Geometry check sheet. Reference: the model listing, model coordinates, mm. Face numbers are marked on the shaded views. A direction names the side the tool comes from. Give positions to 0.01 mm unless a question says otherwise; leave off trailing zeros. Order: outer loops, then holes, each group sorted by start corner. A loop starts at its lowest first (then second) coordinate and runs counter-clockwise, first axis right, second up. Notation, with made-up numbers: (70.25, 83.25) - (77.25, 83.25) arc R28 ccw to (77.25, 105.25) - close; hole circle Ø1 at (6.25, 38.25). An arc over 180 degrees is marked (long way). Put each result on its own line as item: value. Start each with the question number.
```python
from build123d import *

# Parameters (mm, degrees)
F1_DEPTH    = 10
F3_DEPTH    = 1
F4_T1_DEPTH = 100
F4_T4_ANGLE = 180
F4_T6_ANGLE = 180
F6_DEPTH    = 9
F7_R        = 1.1168399156
F8_DEPTH    = 100


# Not quite as in the source:
# - a fillet or chamfer that OpenCascade refuses, or shapes differently, is made with other operations: its cross-section is extruded or revolved along the edge and cut away or added


with BuildPart() as f1:
    # F0 (on Top) → F1 (new body)
    with BuildSketch(Plane.XY):
        with BuildLine():
            Line((48.6515399069, 4.7592671573), (-51.3484600931, 4.7592671573))
            ThreePointArc((-51.3484600931, 4.7592671573), (-61.8484600931, -5.7407328427), (-51.3484600931, -16.2407328427))
            Line((-51.3484600931, -16.2407328427), (48.6515399069, -16.2407328427))
            ThreePointArc((48.6515399069, -16.2407328427), (59.1515399069, -5.7407328427), (48.6515399069, 4.7592671573))
        make_face()
    extrude(amount=F1_DEPTH)

    # F2 (on face) → F3 (join)
    with BuildSketch(Plane.XY.offset(10)):
        with BuildLine():
            Line((48.6515399069, 6.7592671573), (-51.3484600931, 6.7592671573))
            ThreePointArc((-51.3484600931, 6.7592671573), (-63.8484600931, -5.7407328427), (-51.3484600931, -18.2407328427))
            Line((-51.3484600931, -18.2407328427), (48.6515399069, -18.2407328427))
            ThreePointArc((48.6515399069, -18.2407328427), (61.1515399069, -5.7407328427), (48.6515399069, 6.7592671573))
        make_face()
        with BuildLine():
            Line((-51.3484600931, 4.7592671573), (48.6515399069, 4.7592671573))
            ThreePointArc((48.6515399069, 4.7592671573), (59.1515399069, -5.7407328427), (48.6515399069, -16.2407328427))
            Line((48.6515399069, -16.2407328427), (-51.3484600931, -16.2407328427))
            ThreePointArc((-51.3484600931, -16.2407328427), (-61.8484600931, -5.7407328427), (-51.3484600931, 4.7592671573))
        make_face(mode=Mode.SUBTRACT)
        with BuildLine():
            ThreePointArc((48.6515399069, -16.2407328427), (59.1515399069, -5.7407328427), (48.6515399069, 4.7592671573))
            Line((48.6515399069, 4.7592671573), (-51.3484600931, 4.7592671573))
            ThreePointArc((-51.3484600931, 4.7592671573), (-61.8484600931, -5.7407328427), (-51.3484600931, -16.2407328427))
            Line((-51.3484600931, -16.2407328427), (48.6515399069, -16.2407328427))
        make_face()
    extrude(amount=F3_DEPTH)

    # F4: fillet of radius 6 on 4 edges, made by hand

    # F4_s2 → F4_t1 (cut)
    with BuildSketch(Plane.YZ.offset(-51.3484600931)):
        with BuildLine():
            ThreePointArc((6.7592671573, 10), (5.1746931745, 10.7445626465), (3.4426423669, 11))
            Line((3.4426423669, 11), (6.7592671573, 11))
            Line((6.7592671573, 11), (6.7592671573, 10))
        make_face()
        with BuildLine():
            ThreePointArc((-18.2407328427, 10), (-16.6561588599, 10.7445626465), (-14.9241080524, 11))
            Line((-14.9241080524, 11), (-18.2407328427, 11))
            Line((-18.2407328427, 11), (-18.2407328427, 10))
        make_face()
    extrude(amount=F4_T1_DEPTH, mode=Mode.SUBTRACT)

    # F4_s3 → F4_t4 (revolve, cut)
    with BuildSketch(Plane.YZ.offset(48.6515399069)):
        with BuildLine():
            ThreePointArc((-18.2407328427, 10), (-16.6561588599, 10.7445626465), (-14.9241080524, 11))
            Line((-14.9241080524, 11), (-18.2407328427, 11))
            Line((-18.2407328427, 11), (-18.2407328427, 10))
        make_face()
    revolve(axis=Axis((48.6515399069, -5.7407328427, 11), (0, 0, 1)), revolution_arc=F4_T4_ANGLE, mode=Mode.SUBTRACT)

    # F4_s5 → F4_t6 (revolve, cut)
    with BuildSketch(Plane.YZ.offset(-51.3484600931)):
        with BuildLine():
            ThreePointArc((3.4426423669, 11), (5.1746931745, 10.7445626465), (6.7592671573, 10))
            Line((6.7592671573, 10), (6.7592671573, 11))
            Line((6.7592671573, 11), (3.4426423669, 11))
        make_face()
    revolve(axis=Axis((-51.3484600931, -5.7407328427, 11), (0, 0, 1)), revolution_arc=F4_T6_ANGLE, mode=Mode.SUBTRACT)

    # F5 (on face) → F6 (cut)
    with BuildSketch(Plane.XY.offset(11)):
        with BuildLine():
            Line((48.6515399069, 2.4426423669), (-51.3484600931, 2.4426423669))
            ThreePointArc((-51.3484600931, 2.4426423669), (-59.5318353028, -5.7407328427), (-51.3484600931, -13.9241080524))
            Line((-51.3484600931, -13.9241080524), (48.6515399069, -13.9241080524))
            ThreePointArc((48.6515399069, -13.9241080524), (56.8349151165, -5.7407328427), (48.6515399069, 2.4426423669))
        make_face()
    extrude(amount=-F6_DEPTH, mode=Mode.SUBTRACT)

    # F7 (on Right) → F8 (cut, symmetric)
    with BuildSketch(Plane.YZ):
        with Locations((-5.6874994189, 6)):
            Circle(F7_R)
    extrude(amount=F8_DEPTH, both=True, mode=Mode.SUBTRACT)


solid = f1.part
```
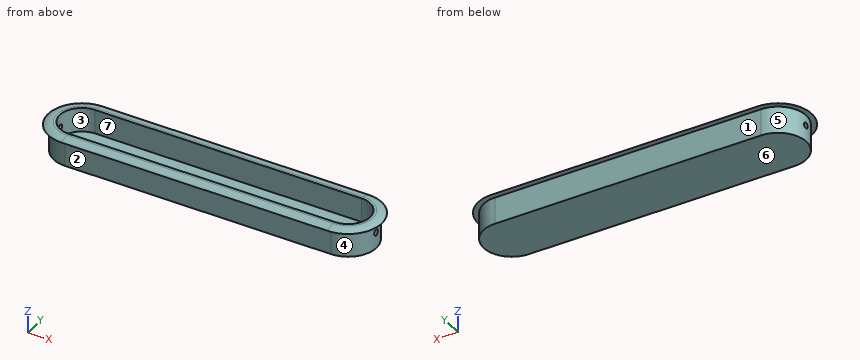
Item 1: Cross-section at A-A (x = 35). Enter the section's corners in (y, z), and give its area (3 significant figures).
Item 2: Release check for a two-part mould opening along Y. For the marked faces 5, 6 and 7 record: +Y half, -Y half, draft (parallel to the pull), parting line (faces both ways), or undercut.
Item 3: Set-up check for the marked faces 1, 2, 3 and 4: record each of +Z, -Z, +X, -X, +Y, -Y from which the full face is reachable in a straight line by a thin tool's end or side.
Item 4: Gauge pin test, flat ends, axial feed: pin 1 Ø6 at (x, z) = (-43, 6.5) entering from +Y; pin 2 Ø13 at (x, y) = (11, -4) entering from +Z; pin 3 Ø2.5 at (y, z) = (-5.69, 6) entering from +X; pin 4 Ø1 at (y, z) = (-12, 5) entering from +X. Record the tip position at first contact, or that the pin passes through.
Item 5: Thickness scan on line 1 along Y through (x, z) = (39, 6.75); line 2 along Z through (x, y) = (-24.5, -0.25); line 3 along X through (y, z) = (-12, 2.75). Record the ranges inside material, lowest first.
Recorded:
1. outline: (-18.24, 10) - (-16.24, 10) - (-16.24, 0) - (4.76, 0) - (4.76, 10) - (6.76, 10) arc R6 ccw to (3.44, 11) - (2.44, 11) - (2.44, 2) - (-13.92, 2) - (-13.92, 11) - (-14.92, 11) arc R6 ccw to start
1. area: 85.6 mm^2
2. face 5: parting line
2. face 6: draft
2. face 7: undercut
3. face 1: -Z, +X, -X, +Y
3. face 2: -Z, +X, -X, -Y
3. face 3: +Z
3. face 4: -Z, +X
4. pin 1: stops at y = 4.76
4. pin 2: stops at z = 11
4. pin 3: stops at x = 59.15
4. pin 4: stops at x = 57.43
5. line 1: y = -16.24 to -13.92, 2.44 to 4.76
5. line 2: z = 0 to 2
5. line 3: x = -59.78 to -56.62, 53.92 to 57.08
